```python
from build123d import *

# Parameters (mm, degrees)
BOSS_EXTRUDE1_DEPTH = 3
SKETCH2_R           = 2.5
BOSS_EXTRUDE2_DEPTH = 25
CUT_EXTRUDE1_REACH  = 46.463
SKETCH5_R           = 3
BOSS_EXTRUDE3_DEPTH = 20
BOSS_EXTRUDE4_DEPTH = 3
SKETCH9_W           = 21
SKETCH9_H           = 21
CUT_EXTRUDE3_DEPTH  = 49
SKETCH10_W          = 21
SKETCH10_H          = 21
CUT_EXTRUDE4_DEPTH  = 49
BOSS_EXTRUDE5_DEPTH = 30
CUT_EXTRUDE5_REACH  = 80.67
SKETCH12_R          = 3
CUT_EXTRUDE6_REACH  = 80.67
SKETCH13_R          = 3
SKETCH14_OUTSIDE_W  = 75.88
SKETCH14_OUTSIDE_H  = 75.88
CUT_EXTRUDE8_DEPTH  = 29


with BuildPart() as part:
    # Sketch1 → Boss-Extrude1 (new body)
    with BuildSketch(Plane(origin=(0, 0, 0), x_dir=(1, 0, 0), z_dir=(0, 1, 0))):
        Polygon((0, -26), (26, -26), (26, 26), (-26, 26), (-26, 0), (0, 0), align=None)
    extrude(amount=BOSS_EXTRUDE1_DEPTH)

    # Sketch2 → Boss-Extrude2 (add)
    with BuildSketch(Plane(origin=(0, 3, 0), x_dir=(1, 0, 0), z_dir=(0, 1, 0))):
        with Locations(Location((13, 13, 0), (0, 0, 90))):
            Circle(SKETCH2_R)
    extrude(amount=BOSS_EXTRUDE2_DEPTH)

    # Sketch5 → Cut-Extrude1 (cut, up to next)
    with BuildSketch(Plane(origin=(0, 3, 0), x_dir=(1, 0, 0), z_dir=(0, 1, 0)), mode=Mode.PRIVATE) as cut_extrude1_sk1:
        with Locations(Location((-13, 13, 0), (0, 0, 270))):
            Circle(SKETCH5_R)
    cut_extrude1_tool1 = extrude(cut_extrude1_sk1.sketch, amount=-CUT_EXTRUDE1_REACH, mode=Mode.PRIVATE) & part.part
    # Sketch5 → Cut-Extrude1 (cut, up to next)
    with BuildSketch(Plane(origin=(0, 3, 0), x_dir=(1, 0, 0), z_dir=(0, 1, 0)), mode=Mode.PRIVATE) as cut_extrude1_sk2:
        with Locations(Location((13, -13, 0), (0, 0, 270))):
            Circle(SKETCH5_R)
    cut_extrude1_tool2 = extrude(cut_extrude1_sk2.sketch, amount=-CUT_EXTRUDE1_REACH, mode=Mode.PRIVATE) & part.part
    add(cut_extrude1_tool1.solids().sort_by_distance((-13, 3, -13))[0], mode=Mode.SUBTRACT)
    add(cut_extrude1_tool2.solids().sort_by_distance((13, 3, 13))[0], mode=Mode.SUBTRACT)

    # Sketch7 → Boss-Extrude3 (add)
    with BuildSketch(Plane.XZ):
        Polygon((26, -26), (26, 26), (0, 26), (0, 0), (-26, 0), (-26, -26), align=None)
        Polygon((23, -23), (23, 23), (3, 23), (3, -3), (-23, -3), (-23, -23), align=None, mode=Mode.SUBTRACT)
    extrude(amount=BOSS_EXTRUDE3_DEPTH)

    # Sketch8 → Boss-Extrude4 (add)
    with BuildSketch(Plane.XZ.offset(20)):
        Polygon((-26, -26), (26, -26), (26, 26), (0, 26), (0, 0), (-26, 0), align=None)
    extrude(amount=BOSS_EXTRUDE4_DEPTH)

    # Sketch9 → Cut-Extrude3 (cut)
    with BuildSketch(Plane.XY.offset(26)):
        with Locations((13, -10)):
            Rectangle(SKETCH9_W, SKETCH9_H)
    extrude(amount=-CUT_EXTRUDE3_DEPTH, mode=Mode.SUBTRACT)

    # Sketch10 → Cut-Extrude4 (cut)
    with BuildSketch(Plane.ZY.offset(26)):
        with Locations((-13, -10)):
            Rectangle(SKETCH10_W, SKETCH10_H)
    extrude(amount=-CUT_EXTRUDE4_DEPTH, mode=Mode.SUBTRACT)

    # Sketch11 → Boss-Extrude5 (add)
    with BuildSketch(Plane.XZ.offset(23)):
        Polygon((-26, 0), (-26, -26), (26, -26), (26, 26), (0, 26), (0, 0), align=None)
    extrude(amount=BOSS_EXTRUDE5_DEPTH)

    # Sketch12 → Cut-Extrude5 (cut, up to next)
    with BuildSketch(Plane(origin=(0, 0, -26), x_dir=(-1, 0, 0), z_dir=(0, 0, -1)), mode=Mode.PRIVATE) as cut_extrude5_sk1:
        with Locations((-13, -10)):
            Circle(SKETCH12_R)
    cut_extrude5_tool1 = extrude(cut_extrude5_sk1.sketch, amount=-CUT_EXTRUDE5_REACH, mode=Mode.PRIVATE) & part.part
    # Sketch12 → Cut-Extrude5 (cut, up to next)
    with BuildSketch(Plane(origin=(0, 0, -26), x_dir=(-1, 0, 0), z_dir=(0, 0, -1)), mode=Mode.PRIVATE) as cut_extrude5_sk2:
        with Locations((13, -10)):
            Circle(SKETCH12_R)
    cut_extrude5_tool2 = extrude(cut_extrude5_sk2.sketch, amount=-CUT_EXTRUDE5_REACH, mode=Mode.PRIVATE) & part.part
    add(cut_extrude5_tool1.solids().sort_by_distance((13, -10, -26))[0], mode=Mode.SUBTRACT)
    add(cut_extrude5_tool2.solids().sort_by_distance((-13, -10, -26))[0], mode=Mode.SUBTRACT)

    # Sketch13 → Cut-Extrude6 (cut, up to next)
    with BuildSketch(Plane(origin=(26, 0, 0), x_dir=(0, 0, -1), z_dir=(1, 0, 0)), mode=Mode.PRIVATE) as cut_extrude6_sk1:
        with Locations((-11.5, -10.917464776)):
            Circle(SKETCH13_R)
    cut_extrude6_tool1 = extrude(cut_extrude6_sk1.sketch, amount=-CUT_EXTRUDE6_REACH, mode=Mode.PRIVATE) & part.part
    # Sketch13 → Cut-Extrude6 (cut, up to next)
    with BuildSketch(Plane(origin=(26, 0, 0), x_dir=(0, 0, -1), z_dir=(1, 0, 0)), mode=Mode.PRIVATE) as cut_extrude6_sk2:
        with Locations((11.5, -10.917464776)):
            Circle(SKETCH13_R)
    cut_extrude6_tool2 = extrude(cut_extrude6_sk2.sketch, amount=-CUT_EXTRUDE6_REACH, mode=Mode.PRIVATE) & part.part
    add(cut_extrude6_tool1.solids().sort_by_distance((26, -10.917465, 11.5))[0], mode=Mode.SUBTRACT)
    add(cut_extrude6_tool2.solids().sort_by_distance((26, -10.917465, -11.5))[0], mode=Mode.SUBTRACT)

    # Sketch14 outside → Cut-Extrude8 (cut)
    # profile 1 of 2: a face of its own
    with BuildSketch(Plane.XZ.offset(53)):
        Rectangle(SKETCH14_OUTSIDE_W, SKETCH14_OUTSIDE_H)
        Polygon((0, 0), (-26, 0), (-26, -26), (26, -26), (26, 26), (0, 26), align=None, mode=Mode.SUBTRACT)
    # profile 2 of 2: a face of its own
    with BuildSketch(Plane.XZ.offset(53)):
        Polygon((5, -5), (-21, -5), (-21, -21), (21, -21), (21, 21), (5, 21), align=None)
    extrude(amount=-CUT_EXTRUDE8_DEPTH, mode=Mode.SUBTRACT)


solid = part.part
```
The model under review builds one solid part; all positions refer to its coordinate system, in mm. A direction names the side the tool comes from. Round coordinates to 2 decimals unless told otherwise and drop trailing zeros. Loops run counter-clockwise (first coordinate to the right, second up) from the corner with the lowest first, then second, coordinate; pieces in that order, holes last. Notation, with made-up numbers: (70, 88) - (101, 88) arc R31 ccw to (101, 112) - close; hole circle Ø7 at (40.25, 12.25). An arc over 180 degrees is marked (long way). Write each question's results on one line, items separated by ' | '. Start each with the question number.
Q1. Draft analysis for pull direction X (two halves, no side actions). For faces 5 (the cylindrical face through (11.2, 1.8, 10.6)), 6 (the cylindrical face through (24.768, -7.943, 11.891)), 7 (the cylindrical face through (14.5, 15.3, -11)), state which applies: pulls with the +X half, pulls with the -X half, needs draft (parallel to the pull), parting line crosses it, or undercut.
Q2. Take a section at A-A on y = -2.5. Give the boundary of the cut face in (x, z).
Q3. Insertion check: P1, Ø3, axis at x = 3, y = -8.5, coming from the +Z side; P2, Ø2, axis at y = -39.5, z = 19, coming from the -X side; P3, Ø5, axis at x = 13, y = -10, coming from the +Z side; P4, Ø12, axis at y = 14, z = -10, coming from the +X side. Each pin has a flat end and moves straight along its axis. Give the tip position at first contact, or say it passes through.
Q4. Take a section at B-B on x = -13. Give the boundary of the cut face in (y, z), plus the area to 3 significant figures.
Q5. Take a section at D-D on z = 20. Give the boundary of the cut face in (x, y).
Q6. Wall thickness on line 1 along Z through (x, y) = (9.5, -42); line 2 along Z through (x, y) = (-1, -36.5); line 3 along Y through (x, z) = (24.2, -11.5): over which ranges is each line inside the solid? List them lowest first. Write a range as [from, to].
Q7. Take a section at C-C on y = -43. Give the boundary of the cut face in (x, z).
Q8. Tool access review of faces 1 (the flat face through (4, 0.5, -5)), 2 (the flat face through (0, -39, -21)), 3 (the flat face through (23.5, -10, 2)), 4 (the flat face through (0, -25, 13)): name each direction out of +Z, -Z, +X, -X, +Y, -Y from which nothing blocks a thin tool from reaching the whole face with its end or side.
Data:
1) face 5: undercut | face 6: needs draft | face 7: parting line crosses it
2) outline: (-26, -26) - (26, -26) - (26, 26) - (23.5, 26) - (23.5, -23) - (23, -23) - (23, -23.5) - (-26, -23.5) - close; (-26, -2.5) - (2.5, -2.5) - (2.5, 26) - (0, 26) - (0, 0) - (-26, 0) - close
3) P1: stops at z = 26 | P2: stops at x = 0 | P3: passes through | P4: stops at x = 15.5
4) outline: (-53, -26) - (-13, -26) - (-13, -23.5) - (-20.5, -23.5) - (-20.5, -2.5) - (0.5, -2.5) - (0.5, -10) - (3, -10) - (3, 0) - (-53, 0) - (-53, -5) - (-24, -5) - (-24, -21) - (-53, -21) - close; (-7, -26) - (3, -26) - (3, -16) - (0.5, -16) - (0.5, -23.5) - (-7, -23.5) - close | area: 521 mm²
5) outline: (0, -53) - (5, -53) - (5, -24) - (21, -24) - (21, -53) - (26, -53) - (26, 3) - (0, 3) - close; hole (2.5, -20.5) - (23.5, -20.5) - (23.5, 0.5) - (2.5, 0.5) - close
6) line 1: z = [-26, -21], [21, 26] | line 2: z = [-26, -21], [-5, 0] | line 3: y = [-53, -13.92], [-7.92, 3]
7) outline: (-26, -26) - (26, -26) - (26, 26) - (0, 26) - (0, 0) - (-26, 0) - close; hole (-21, -21) - (21, -21) - (21, 21) - (5, 21) - (5, -5) - (-21, -5) - close
8) face 1: none | face 2: -Y | face 3: +Z | face 4: +Z, -X, +Y, -Y
